Verification items for the finished model (mm, model axes). A direction names the side the tool comes from. Give positions to 0.01 mm unless a question says otherwise; leave off trailing zeros. Loops run counter-clockwise (first coordinate to the right, second up) from the corner with the lowest first, then second, coordinate; pieces in that order, holes last. Notation, with made-up numbers: (14, 25.5) -> (59, 25.5) arc R17 ccw to (59, 54.5) -> close; hole circle Ø11 at (83, 58). An arc over 180 degrees is marked (long way). Answer in a Markdown table with one row per item. Add a question column.
Q1. Section check A-A on y = 4.5. Enter the section's corners in (x, z), and give its area (3 significant figures).
Q2. Section check C-C on y = -1. Enter the section's corners in (x, z) (3 decimals).
Q3. Material ranges on probe 1 along X at (y, z) = (4.25, 26); probe 2 along X at (y, z) = (2.75, 5); probe 3 along Y at (x, z) = (-1.25, 21.5), recorded low to high.
Q4. Section check D-D on x = 0. Enter the section's corners in (y, z), and give its area (4 significant figures).
Q5. Release check for a two-part mould opening along X. For faces 6 (the face through (0, 1, -31.75)), 7 (the face through (2.375, -1.726, -19.012)), 8 (the face through (-1, -2, -19)), 9 (the face through (-2.375, -1.726, 19.012)) record: pulls with the +X half, pulls with the -X half, needs draft (parallel to the pull), parting line crosses it, or undercut.
Q6. Set-up check for faces 1 (the face through (-1, 4, 0)), 2 (the face through (1.32, 3.89, 28.51)), 3 (the face through (2.375, -1.726, 19.088)), 4 (the face through (1.33, 3.89, -28.59)), 5 (the face through (1, -2, -19)): record each of +Z, -Z, +X, -X, +Y, -Y from which the full face is reachable in a straight line by a thin tool's end or side.
Q7. Section check B-B on z = 15.5. Enter the section's corners in (x, y), and give its area (3 significant figures).
Q8. Gauge pin test, flat ends, axial feed: P1, Ø5, axis at y = -3.5, z = 16, coming from the +X side; P2, Ø1.3, axis at y = -3.5, z = -19.5, coming from the +X side (3 decimals); P3, Ø1.3, axis at y = -3.5, z = 19, coming from the -X side (3 decimals); P4, Ø3, axis at x = -1.5, y = 3.5, coming from the +Z side. Record the tip position at first contact, or that the pin passes through.
Autodesk Inventor part; units mm, degrees
ref_plane "YZ Plane" through (0, 0, 0) normal (1, 0, 0) x (0, 1, 0)
ref_plane "XZ Plane" through (0, 0, 0) normal (0, 1, 0) x (-1, 0, 0)
ref_plane "XY Plane" through (0, 0, 0) normal (0, 0, 1) x (1, 0, 0)
sketch "Esquisse1" plane through (0, 0, 0) normal (0, 1, 0) x (-1, 0, 0)
  line L0 (3.2, 31.75) -> (-3.2, 31.75)
  line L1 (-3.2, 31.75) -> (-3.2, -31.75)
  line L2 (-3.2, -31.75) -> (3.2, -31.75)
  line L3 (3.2, -31.75) -> (3.2, 31.75)
  point P0 (0, 0)
  dimension "d0" = 63.5
  dimension "d1" = 6.4
  dimension "d2" = 3.2
  dimension "d3" = 31.75
extrude "Extrusion1" add sketch "Esquisse1" along normal blind 6.4
sketch "Esquisse2" plane through (0, 6.4, 0) normal (0, 1, 0) x (1, 0, 0)
  line L0 (-3.2, -31.75) -> (3.2, -31.75)
  line L1 (-1.65, -31.75) -> (-1, -25.35)
  line L2 (-1, -25.35) -> (-1, 25.35)
  line L3 (-1, 25.35) -> (-1.65, 31.75)
  line L4 (3.2, 31.75) -> (-3.2, 31.75)
  line L5 (-1.65, 31.75) -> (1.65, 31.75)
  line L6 (1.65, 31.75) -> (1, 25.35)
  line L7 (1, 25.35) -> (1, -25.35)
  line L8 (1, -25.35) -> (1.65, -31.75)
  line L9 (1.65, -31.75) -> (-1.65, -31.75)
  point P0 (0, 0)
  dimension "d6" = 3.3
  dimension "d7" = 3.3
  dimension "d8" = 1.65
  dimension "d9" = 1.65
  dimension "d10" = 2
  dimension "d11" = 1
  dimension "d12" = 6.4
  dimension "d13" = 6.4
  dimension "d14" = 6.4
  dimension "d15" = 6.4
extrude "Extrusion2" cut sketch "Esquisse2" against normal blind 5.1
sketch "Esquisse3" plane through (0, 0, 0) normal (0, -1, 0) x (1, 0, 0)
  circle A0 centre (0, 19.05) radius 2.375
  circle A1 centre (0, -19.05) radius 2.375
  line L0 (-3.2, -31.75) -> (-3.2, 31.75)
  line L1 (3.2, 31.75) -> (3.2, -31.75)
  point P0 (0, 0)
  dimension "d18" = 4.75
  dimension "d19" = 19.05
  dimension "d20" = 38.1
  dimension "d21" = 4.75
  dimension "d22" = 6.4
  dimension "d23" = 3.2
  dimension "d24" = 3.2
extrude "Extrusion3" add sketch "Esquisse3" along normal blind 4.8
sketch "Esquisse4" plane through (0, -4.8, 19.05) normal (0, -1, 0) x (1, 0, 0)
  line L0 (-1, 6.3) -> (-1, -44.4)
  line L1 (1, 3.95) -> (-1, 3.95)
  line L2 (-1, 3.95) -> (-1, -4.05)
  line L3 (-1, -4.05) -> (1, -4.05)
  line L4 (1, -4.05) -> (1, 3.95)
  line L5 (1, -34.05) -> (-1, -34.05)
  line L6 (-1, -34.05) -> (-1, -42.05)
  line L7 (-1, -42.05) -> (1, -42.05)
  line L8 (1, -42.05) -> (1, -34.05)
  point P0 (0, -19.05)
  point P1 (-1, 3.95)
  dimension "d27" = 2
  dimension "d28" = 15
  dimension "d29" = 15
  dimension "d30" = 8
  dimension "d31" = 8
extrude "Extrusion4" cut sketch "Esquisse4" against normal blind 4.8
chamfer "Chanfrein1" distance 1.3 angle 45 2 edges at (2.375, -4.8, 19.05) (-2.375, -4.8, 19.05)
chamfer "Chanfrein2" distance 1.3 angle 45 2 edges at (-2.375, -4.8, -19.05) (2.375, -4.8, -19.05)
equation "\"d7\" = d6"
equation "\"d13\" = d12"
equation "\"d14\" = d12"
equation "\"d15\" = d12"
equation "\"d21\" = d18"
equation "\"d23\" = 0.5 * d22"
equation "\"d24\" = d23"
properties part number "RDC-250" material "Nylon 6/6"
Taken from the geometry:
| question | item | result |
|---|---|---|
| 1 | outline | (-3.2, -31.75) -> (-1.65, -31.75) -> (-1, -25.35) -> (-1, 25.35) -> (-1.65, 31.75) -> (-3.2, 31.75) -> close; (1, -25.35) -> (1.65, -31.75) -> (3.2, -31.75) -> (3.2, 31.75) -> (1.65, 31.75) -> (1, 25.35) -> close |
| 1 | area | 271 mm² |
| 2 | outline | (-1, -21.204) -> (-1, -16.896) arc R2.375 ccw to start; (-1, 16.896) -> (-1, 21.204) arc R2.375 ccw to start; (1, -21.204) arc R2.375 ccw to (1, -16.896) -> close; (1, 16.896) arc R2.375 ccw to (1, 21.204) -> close |
| 3 | probe 1 | x = -3.2 to -1.07, 1.07 to 3.2 |
| 3 | probe 2 | x = -3.2 to -1, 1 to 3.2 |
| 3 | probe 3 | y = 0 to 6.4 |
| 4 | outline | (0, -31.75) -> (1.3, -31.75) -> (1.3, 31.75) -> (0, 31.75) -> close |
| 4 | area | 82.55 mm² |
| 5 | face 6 | needs draft |
| 5 | face 7 | pulls with the +X half |
| 5 | face 8 | undercut |
| 5 | face 9 | pulls with the -X half |
| 6 | face 1 | +Z, -Z, +Y |
| 6 | face 2 | +Z, +Y |
| 6 | face 3 | +X, -Y |
| 6 | face 4 | -Z, +Y |
| 6 | face 5 | +Z, -Z, -Y |
| 7 | outline | (-3.2, 0) -> (3.2, 0) -> (3.2, 6.4) -> (1, 6.4) -> (1, 1.3) -> (-1, 1.3) -> (-1, 6.4) -> (-3.2, 6.4) -> close |
| 7 | area | 30.8 mm² |
| 8 | P1 | stops at x = 2.31 |
| 8 | P2 | stops at x = 2.375 |
| 8 | P3 | stops at x = -2.375 |
| 8 | P4 | stops at z = 31.75 |
